The model under review builds one solid part; all positions refer to its coordinate system, in mm. Face numbers are marked on the shaded views. A direction names the side the tool comes from. Give positions to 0.01 mm unless a question says otherwise; leave off trailing zeros. Loops run counter-clockwise (first coordinate to the right, second up) from the corner with the lowest first, then second, coordinate; pieces in that order, holes last. Notation, with made-up numbers: M 43,-25 L 92,-25 A21 cw 92,-5 Z; hole C 0,23 d3. An arc over 180 degrees is marked long. Return JSON: item names as keys, results as strings. Group by question number.
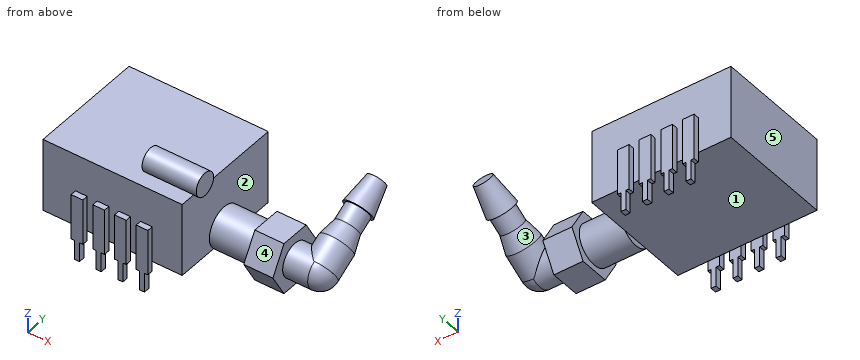
```python
from build123d import *

# Parameters (mm, degrees)
ESQUISSE1_W                = 16.7
ESQUISSE1_H                = 13.9
EXTRUSION1_DEPTH           = 8.8
EXTRUSION2_DEPTH           = 0.5
EXTRUSION2_DEPTH_BACK      = 6
ESQUISSE2_R                = 1.4
ESQUISSE3_R                = 2.4
EXTRUSION3_DEPTH           = 5
EXTRUSION4_DEPTH           = 3.5
ESQUISSE5_R                = 2
EXTRUSION5_DEPTH           = 5
CONG_1_R                   = 2
ESQUISSE6_R                = 2
EXTRUSION6_DEPTH           = 3
EXTRUSION6_OTHER_WAY_DEPTH = 2
EXTRUSION6_OTHER_WAY_TAPER = 15
ESQUISSE7_R                = 1.464101615
EXTRUSION7_DEPTH           = 2
ESQUISSE8_R                = 1.75
EXTRUSION8_DEPTH           = 3.5
EXTRUSION8_TAPER           = 10
EXTRUSION9_DEPTH           = 0.7
EXTRUSION10_DEPTH          = 0.7


with BuildPart() as part:
    # Esquisse1 → Extrusion1 (new body)
    with BuildSketch(Plane.XY):
        with Locations((0.361659441, 0.162554307)):
            Rectangle(ESQUISSE1_W, ESQUISSE1_H)
    extrude(amount=-EXTRUSION1_DEPTH)

    # Esquisse2 → Extrusion2 (add, two sides: drawn at the far end of the back side and taken through both)
    with BuildSketch(Plane(origin=(8.711659441, 0, 0), x_dir=(0, 0, -1), z_dir=(1, 0, 0)).offset(-EXTRUSION2_DEPTH_BACK)):
        with Locations((-0.8, -3.787445693)):
            Circle(ESQUISSE2_R)
    extrude(amount=EXTRUSION2_DEPTH + EXTRUSION2_DEPTH_BACK)

    # Esquisse3 → Extrusion3 (add)
    with BuildSketch(Plane(origin=(8.711659441, 0, 0), x_dir=(0, 0, -1), z_dir=(1, 0, 0))):
        with Locations(Location((7.1, 0, 0), (0, 0, 315.099472039))):
            Circle(ESQUISSE3_R)
    extrude(amount=EXTRUSION3_DEPTH)

    # Esquisse4 → Extrusion4 (add)
    with BuildSketch(Plane(origin=(13.711659441, 0, 0), x_dir=(0, 0, -1), z_dir=(1, 0, 0))):
        Polygon((10.198101751, -1.793069678), (10.201894768, 1.786499981), (7.103793016, 3.579569659), (4.001898249, 1.793069678), (3.998105232, -1.786499981), (7.096206984, -3.579569659), align=None)
    extrude(amount=EXTRUSION4_DEPTH)

    # Esquisse5 → Extrusion5 (add)
    with BuildSketch(Plane(origin=(17.211659441, 0, 0), x_dir=(0, 0, -1), z_dir=(1, 0, 0))):
        with Locations(Location((7.1, 0, 0), (0, 0, 180))):
            Circle(ESQUISSE5_R)
    extrude(amount=EXTRUSION5_DEPTH)

    # Congé1
    cong_1_edges = [part.edges().sort_by_distance(p)[0] for p in [
        (22.211659441, 0, -9.1),
    ]]
    fillet(cong_1_edges, radius=CONG_1_R)

    # Esquisse6 → Extrusion6 (add)
    with BuildSketch(Plane(origin=(0, -0.384301931, -0.221334199), x_dir=(-1, 0, 0), z_dir=(0, 0.866554731886771, 0.4990820540198241))):
        with Locations(Location((-20.211659441, -6.152538596, 0), (0, 0, 90))):
            Circle(ESQUISSE6_R)
    extrude(amount=-EXTRUSION6_DEPTH)

    # Esquisse6 → Extrusion6 other way (add)
    with BuildSketch(Plane(origin=(0, -0.384301931, -0.221334199), x_dir=(-1, 0, 0), z_dir=(0, 0.866554731886771, 0.4990820540198241))):
        with Locations(Location((-20.211659441, -6.152538596, 0), (0, 0, 90))):
            Circle(ESQUISSE6_R)
    extrude(amount=EXTRUSION6_OTHER_WAY_DEPTH, taper=EXTRUSION6_OTHER_WAY_TAPER)

    # Esquisse7 → Extrusion7 (add)
    with BuildSketch(Plane(origin=(0, 1.348807532, 0.776829909), x_dir=(-1, 0, 0), z_dir=(0, 0.866554731886771, 0.4990820540198242))):
        with Locations(Location((-20.211659441, -6.152538596, 0), (0, 0, 90))):
            Circle(ESQUISSE7_R)
    extrude(amount=EXTRUSION7_DEPTH)

    # Esquisse8 → Extrusion8 (add)
    with BuildSketch(Plane(origin=(0, 3.081916996, 1.774994017), x_dir=(-1, 0, 0), z_dir=(0, 0.8665547318867707, 0.4990820540198243))):
        with Locations((-20.211659441, -6.152538596)):
            Circle(ESQUISSE8_R)
    extrude(amount=EXTRUSION8_DEPTH, taper=EXTRUSION8_TAPER)

    # Esquisse9 → Extrusion9 (add)
    with BuildSketch(Plane.XZ.offset(6.787445693)):
        Polygon((5.111659441, -4.5), (5.111659441, -10), (4.711659441, -10), (4.711659441, -12.342565152), (4.111659441, -12.342565152), (4.111659441, -10), (3.711659441, -10), (3.711659441, -4.5), align=None)
        Polygon((2.511659441, -4.5), (2.511659441, -10), (2.111659441, -10), (2.111659441, -12.342565152), (1.511659441, -12.342565152), (1.511659441, -10), (1.111659441, -10), (1.111659441, -4.5), align=None)
        Polygon((-0.088340559, -4.5), (-0.088340559, -10), (-0.488340559, -10), (-0.488340559, -12.342565152), (-1.088340559, -12.342565152), (-1.088340559, -10), (-1.488340559, -10), (-1.488340559, -4.5), align=None)
        Polygon((-2.688340559, -4.5), (-2.688340559, -10), (-3.088340559, -10), (-3.088340559, -12.342565152), (-3.688340559, -12.342565152), (-3.688340559, -10), (-4.088340559, -10), (-4.088340559, -4.5), align=None)
    extrude(amount=EXTRUSION9_DEPTH)

    # Esquisse10 → Extrusion10 (add)
    with BuildSketch(Plane(origin=(0, 7.112554307, 0), x_dir=(-1, 0, 0), z_dir=(0, 1, 0))):
        Polygon((0.088340559, -4.5), (0.088340559, -10), (0.488340559, -10), (0.488340559, -12.342565152), (1.088340559, -12.342565152), (1.088340559, -10), (1.488340559, -10), (1.488340559, -4.5), align=None)
        Polygon((-2.511659441, -10), (-2.111659441, -10), (-2.111659441, -12.342565152), (-1.511659441, -12.342565152), (-1.511659441, -10), (-1.111659441, -10), (-1.111659441, -4.5), (-2.511659441, -4.5), align=None)
        Polygon((-4.711659441, -10), (-4.711659441, -12.342565152), (-4.111659441, -12.342565152), (-4.111659441, -10), (-3.711659441, -10), (-3.711659441, -4.5), (-5.111659441, -4.5), (-5.111659441, -10), align=None)
        Polygon((2.688340559, -4.5), (2.688340559, -10), (3.088340559, -10), (3.088340559, -12.342565152), (3.688340559, -12.342565152), (3.688340559, -10), (4.088340559, -10), (4.088340559, -4.5), align=None)
    extrude(amount=EXTRUSION10_DEPTH)


solid = part.part
```
(1) Add section D-D (x = 5.5). Write out the cut boundary in (y, z), and give its area (3 significant figures).
(2) For the marked faces 1 and 2, list the 3-axis set-ups (+Z, -Z, +X, -X, +Y, -Y) from which the entire face can be reached by the end or side of a thin tool; tool diameter is ignored.
(3) Add section A-A (x = 16). Write out the cut boundary in (y, z).
(4) Add section B-B (y = 2.75). Count the separate pieces of the cut face and the enclosed holes in it, and give its area (3 significant figures).
(5) Add section C-C (z = 0.8). Write out the cut boundary in (x, y), and give its area (3 significant figures).
(6) For pin 1 (1 mm diameter, centred on y = -2, z = -10, fed in from +X); pin 2 (1.5 mm diameter, centred on x = -1, z = -7, fed in from +Y); pin 3 (0.6 mm diameter, centred on y = -7, z = -11, fed in from +X), all flat-tipped, find the tip position at first contact; note any pin that passes through.
(7) Mouldability with a two-part tool opening along X and no side actions: class the marked faces 3, 4 and 5 as released by +X, released by -X, zero draft, split by the parting line, or undercut.
(8) For probe 1 along X at (y, z) = (6, -0.75); probe 2 along Y at (x, z) = (5, -3); probe 3 along Z at (x, y) = (-1.5, 1), list the stretches that pass through material, from the lowest coordinate up.
Verdict:
{
 "1": {"outline": "M -6.79,-8.8 L 7.11,-8.8 L 7.11,0 L -2.64,0 A1.4 ccw long -4.94,0 L -6.79,0 Z", "area": "128 mm²"},
 "2": {"face 1": "-Z, -X", "face 2": "none"},
 "3": {"outline": "M -3.58,-7.1 L -1.79,-10.2 L 1.79,-10.2 L 3.58,-7.1 L 1.79,-4 L -1.79,-4 Z"},
 "4": {"separate pieces": "3", "enclosed holes": "0", "area": "170 mm²"},
 "5": {"outline": "M 2.71,-5.19 L 9.21,-5.19 L 9.21,-2.39 L 2.71,-2.39 Z", "area": "18.2 mm²"},
 "6": {"pin 1": "stops at x = 17.21", "pin 2": "stops at y = 7.81", "pin 3": "stops at x = 4.71"},
 "7": {"face 3": "undercut", "face 4": "zero draft", "face 5": "released by -X"},
 "8": {"probe 1": "x = -7.99 to 8.71", "probe 2": "y = -6.79 to 7.11", "probe 3": "z = -8.8 to 0"}
}
